The model under review builds one solid part; all positions refer to its coordinate system, in mm. Face numbers are marked on the shaded views. A direction names the side the tool comes from. Round coordinates to 2 decimals unless told otherwise and drop trailing zeros. Order: outer loops, then holes, each group sorted by start corner. A loop starts at its lowest first (then second) coordinate and runs counter-clockwise, first axis right, second up. Notation, with made-up numbers: M 82.5,48.25 L 117.5,48.25 A20 ccw 117.5,54.25 Z; hole C -29.5,-10 d1. An arc over 180 degrees is marked long. One line per item, written item: value. Start each with the question number.
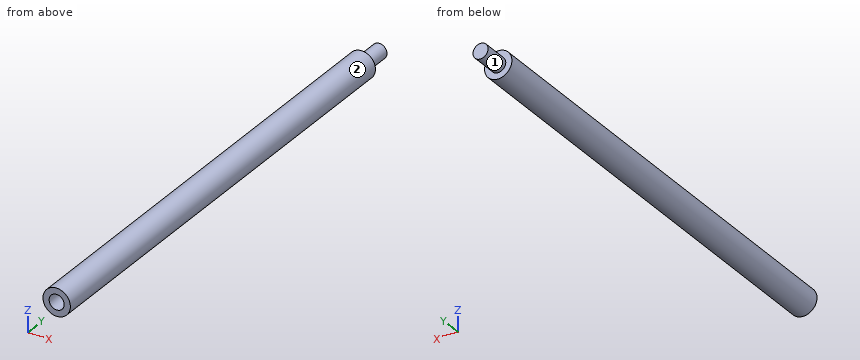
from build123d import *

# Parameters (mm, degrees)
SKETCH1_R                       = 3.175
BOSS_EXTRUDE1_DEPTH             = 109.728
F_6_32_TAPPED_HOLE1_D           = 2.7051
F_6_32_TAPPED_HOLE1_DEPTH       = 9.398
F_6_32_TAPPED_HOLE1_CBORE_D     = 3.5052
F_6_32_TAPPED_HOLE1_CBORE_DEPTH = 7.112
F_6_32_TAPPED_HOLE1_TIP         = 0.81269403
SKETCH4_R                       = 1.7526
BOSS_EXTRUDE2_DEPTH             = 6.35


with BuildPart() as part:
    # Sketch1 → Boss-Extrude1 (new body)
    with BuildSketch(Plane(origin=(0, 0, 0), x_dir=(1, 0, 0), z_dir=(0, 1, 0))):
        Circle(SKETCH1_R)
    extrude(amount=BOSS_EXTRUDE1_DEPTH)

    # #6-32 Tapped Hole1
    with Locations(Plane(origin=(0, 0, 0), x_dir=(-1, 0, 0), z_dir=(0, -1, 0))):
        with Locations((0, 0)):
            CounterBoreHole(F_6_32_TAPPED_HOLE1_D / 2, F_6_32_TAPPED_HOLE1_CBORE_D / 2, F_6_32_TAPPED_HOLE1_CBORE_DEPTH, depth=F_6_32_TAPPED_HOLE1_DEPTH)
            with Locations((0, 0, -(F_6_32_TAPPED_HOLE1_DEPTH + F_6_32_TAPPED_HOLE1_TIP / 2))):  # 118° drill point
                Cone(0, F_6_32_TAPPED_HOLE1_D / 2, F_6_32_TAPPED_HOLE1_TIP, mode=Mode.SUBTRACT)

    # Sketch4 → Boss-Extrude2 (add)
    with BuildSketch(Plane(origin=(0, 109.728, 0), x_dir=(1, 0, 0), z_dir=(0, 1, 0))):
        Circle(SKETCH4_R)
    extrude(amount=BOSS_EXTRUDE2_DEPTH)


solid = part.part
Item 1: Machinability: for the marked faces 1 and 2, which of the approach directions +Z, -Z, +X, -X, +Y, -Y give a long, thin tool a straight path to every point of the face, cutting with its end or side? Answer none if there is none.
Item 2: Clearance check with flat-ended pins moving along their axes: P1, Ø2, axis at y = 99, z = 2, coming from the +X side; P2, Ø1.1, axis at x = 0, z = 0.5, coming from the -Y side. State where each tip first meets the part, or that it passes through.
Item 3: Consider section A-A, the plane y = 70.5. Give the boundary of the cut face in (x, z) (3 decimals), then the cut area to 3 significant figures.
Item 4: Wall thickness on L1, parallel to Z at x = 0, y = 8.55 (3 decimals); L2, parallel to Z at x = 0, y = 3.75 (3 decimals); L3, parallel to Y at x = 1.5, z = -2.25: over which ranges is each line inside the solid? List them lowest first.
Computed:
1. face 1: +Y
1. face 2: +Y, -Y
2. P1: stops at x = 3.01
2. P2: stops at y = 9.58
3. outline: C 0,0 d6.35
3. area: 31.7 mm^2
4. L1: z = -3.175 to -1.353, 1.353 to 3.175
4. L2: z = -3.175 to -1.753, 1.753 to 3.175
4. L3: y = 0 to 109.73
